Part print with two shaded views. Sizes in mm from the minimum x, y, z corner. A direction names the side the tool comes from. Round coordinates to 2 decimals unless told otherwise and drop trailing zeros. Order: outer loops, then holes, each group sorted by start corner. A loop starts at its lowest first (then second) coordinate and runs counter-clockwise, first axis right, second up. Notation, with made-up numbers: (32, 88.25) -> (74, 88.25) arc R13 ccw to (74, 108.25) -> close; hole circle Ø11 at (-7.75, -27.75). An arc over 180 degrees is marked (long way). Answer as a JSON object with one key per item and string values.
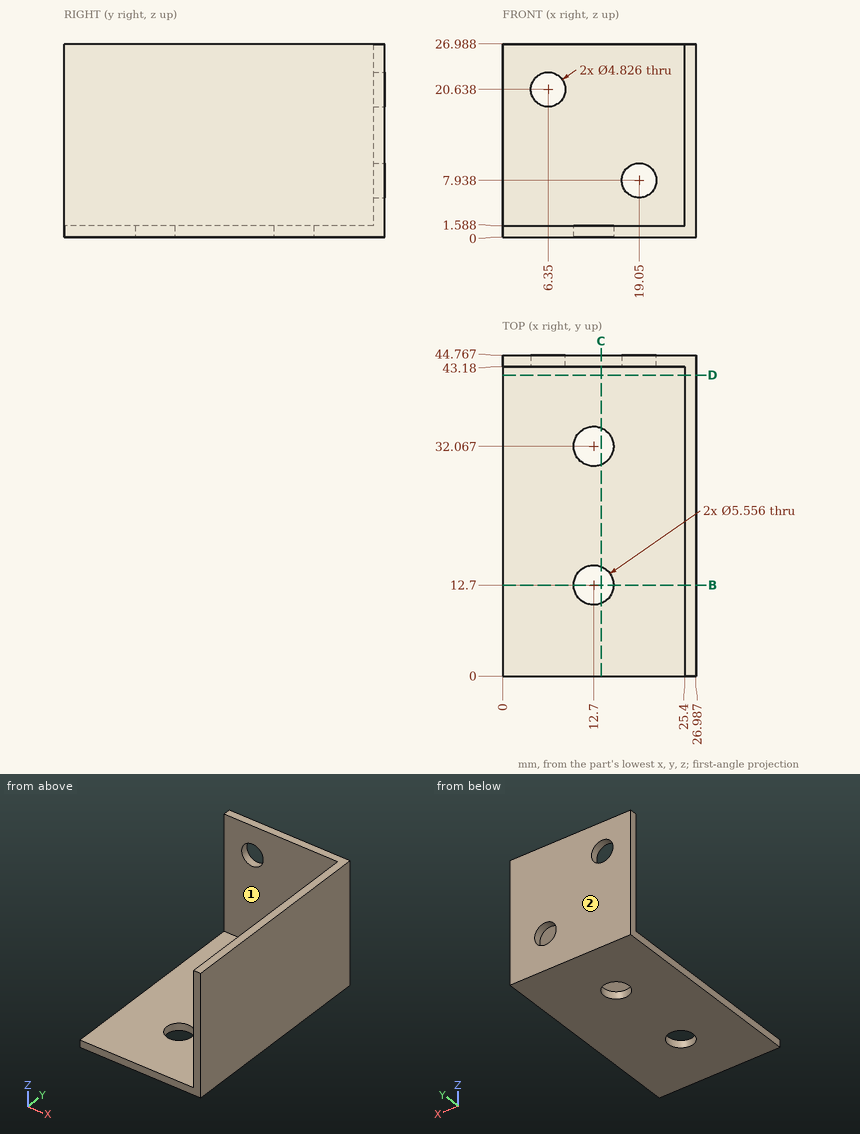
1) Cut at B-B, the plane y = 12.7. Give the cut face in (x, z).
Checked values:
{"outline": "(0, 0) -> (9.92, 0) -> (9.92, 1.59) -> (0, 1.59) -> close; (15.48, 0) -> (26.99, 0) -> (26.99, 26.99) -> (25.4, 26.99) -> (25.4, 1.59) -> (15.48, 1.59) -> close"}
2) Probe L1, parallel to Y at x = 10.5, z = 9; L2, parallel to Z at x = 24, y = 32; L3, parallel to X at y = 9, z = 18.5. List the from-to ranges inside material, lowest first. Write a range as from..to.
Checked values:
{"L1": "y = 43.18..44.77", "L2": "z = 0..1.59", "L3": "x = 25.4..26.99"}
3) Cut at C-C, the plane x = 13.75. Give the cut face in (y, z) (1 decimal).
Checked values:
{"outline": "(0, 0) -> (10.1, 0) -> (10.1, 1.6) -> (0, 1.6) -> close; (15.3, 0) -> (29.5, 0) -> (29.5, 1.6) -> (15.3, 1.6) -> close; (34.6, 0) -> (44.8, 0) -> (44.8, 27) -> (43.2, 27) -> (43.2, 1.6) -> (34.6, 1.6) -> close"}
4) Cut at D-D, the plane y = 42. Give the cut face in (x, z).
Checked values:
{"outline": "(0, 0) -> (26.99, 0) -> (26.99, 26.99) -> (25.4, 26.99) -> (25.4, 1.59) -> (0, 1.59) -> close"}
5) Which spindle directions (+Z, -Z, +X, -X, +Y, -Y) get a long thin tool onto all of the face, cutting with end or side? Do the marked faces 1 and 2. Say none if no direction does.
Checked values:
{"face 1": "+Z, -X, -Y", "face 2": "+Z, -Z, +X, -X, +Y"}
6) Flat gauge pins, fed straight in: pin 1 Ø3 at (x, z) = (6.35, 20.64) entering from +Y; pin 2 Ø1.5 at (x, y) = (7, 25) entering from +Z; pin 3 Ø1.5 at (x, y) = (11.5, 15) entering from -Z; pin 4 Ø7.5 at (x, z) = (7, 10) entering from -Y. Where does each tip first touch, or does it go through?
Checked values:
{"pin 1": "passes through", "pin 2": "stops at z = 1.59", "pin 3": "stops at z = 0", "pin 4": "stops at y = 43.18"}
